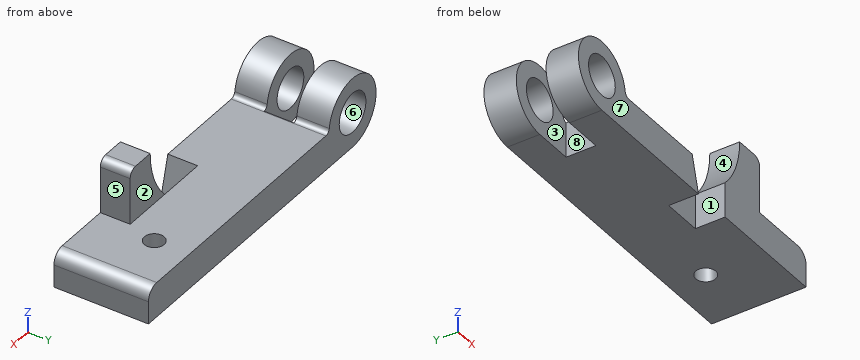
from build123d import *

# Parameters (mm, degrees)
F0_R          = 12.7
F1_DEPTH      = 30.1625
F2_R          = 6.35
F2_W          = 50.010991877
F2_H          = 18.9992
F3_DEPTH      = 22.353
F3_DEPTH_BACK = 25.4
F5_DEPTH      = 19.05
F7_DEPTH      = 19.05
F8_R          = 5.08
F9_R          = 7.874
F10_R         = 3.302


with BuildPart() as f1:
    # F0 (on Front) → F1 (new body, symmetric)
    with BuildSketch(Plane.XZ):
        with BuildLine():
            Line((194.2084, 0), (22.352, 0))
            ThreePointArc((22.352, 0), (-15.8052507731, 15.8052507731), (0, -22.352))
            Line((0, -22.352), (194.2084, -22.352))
            Line((194.2084, -22.352), (194.2084, 0))
        make_face()
        Circle(F0_R, mode=Mode.SUBTRACT)
    extrude(amount=F1_DEPTH, both=True)

    # F2 (on Top) → F3 (cut, two sides)
    with BuildSketch(Plane.XY) as f3_sk:
        with Locations((155.3464, 7.8105)):
            Circle(F2_R)
        Rectangle(F2_W, F2_H)
    extrude(amount=-F3_DEPTH, mode=Mode.SUBTRACT)
    extrude(f3_sk.sketch, amount=F3_DEPTH_BACK, mode=Mode.SUBTRACT)

    # F4 (on face) → F5 (cut)
    with BuildSketch(Plane.XZ.offset(30.1625)):
        Polygon((117.2464, -22.352), (117.2464, 0), (85.852, 0), (91.8464, -22.352), align=None)
    extrude(amount=-F5_DEPTH, mode=Mode.SUBTRACT)

    # F6 (on face) → F7 (join)
    with BuildSketch(Plane.XZ.offset(30.1625)):
        with BuildLine():
            Line((117.2464, 0), (150.0886, 0))
            Line((150.0886, 0), (150.0886, 34.798))
            Line((150.0886, 34.798), (131.0386, 34.798))
            ThreePointArc((131.0386, 34.798), (127.4644153616, 16.0823576341), (117.2464, 0))
        make_face()
    extrude(amount=-F7_DEPTH)

    # F8
    f8_edges = [f1.edges().sort_by_distance(p)[0] for p in [
        (150.0886, -20.6375, 34.798),
    ]]
    fillet(f8_edges, radius=F8_R)

    # F9
    f9_edges = [f1.edges().sort_by_distance(p)[0] for p in [
        (194.2084, 0, 0),
    ]]
    fillet(f9_edges, radius=F9_R)

    # F10
    f10_edges = [f1.edges().sort_by_distance(p)[0] for p in [
        (22.352, -19.83105, 0),
    ]]
    fillet(f10_edges, radius=F10_R)


solid = f1.part
The listing builds one solid part. Answer for the finished solid, in the listing's coordinates (mm). Face numbers are marked on the shaded views. A direction names the side the tool comes from. Round coordinates to 2 decimals unless told otherwise and drop trailing zeros. Write each loop counter-clockwise with the first axis right and the second up, starting at its lowest first coordinate (ties: lowest second). Pieces come first, ordered by that corner, then holes. Notation, with made-up numbers: (75.5, 64) - (130.5, 64) arc R20 cw to (130.5, 97) - close; hole circle Ø2 at (65, 34.25). An arc over 180 degrees is marked (long way). Use a Markdown table: item, result. Add a question column.
1. A tool of negligible diameter and unlimited length cuts with its end or side. For the marked faces 1, 2, 3, 4 and 5, from which of +Z, -Z, +X, -X, +Y, -Y can it reach the whole face along a straight path? Write none if from no direction.
2. The part is cut by section A-A (z = -3). Write down the section's boundary in (x, y).
3. For a pull along Y with two mould halves and no side action, classify the marked faces 6, 7 and 8 as +Y half, -Y half, draft (parallel to the pull), parting line (faces both ways), or undercut.
4. The part is cut by section D-D (x = 155). Write down the section's boundary in (y, z), and give its area (3 significant figures).
5. The part is cut by section B-B (y = 26). Write down the section's boundary in (x, z), and give its area (3 significant figures).
6. The part is cut by section C-C (z = 16). Write down the section's boundary in (x, y), and give its area (3 significant figures).
7. Flat-ended cylindrical pins translate along their axes: P1, Ø1, axis at x = 62, y = -15, coming from the +Z side; P2, Ø5.5, axis at y = -22.5, z = -11, coming from the -X side; P3, Ø18, axis at x = 97, z = -13, coming from the -Y side; P4, Ø15, axis at y = 3.5, z = -11.5, coming from the -X side. Find the tip coordinate at first contact, or state that the pin passes through.
8. Consider line 1 (Z direction, x = 0, y = -14.5); line 2 (Y direction, x = 149, z = 13); line 3 (Y direction, x = 91, z = -3). Determine where each line is inside the solid, lowest interval first.
Reported:
| question | item | result |
|---|---|---|
| 1 | face 1 | +Z, -Z, -Y |
| 1 | face 2 | +Z, +X, +Y |
| 1 | face 3 | +Z, -Z, -X |
| 1 | face 4 | +Z, +Y, -Y |
| 1 | face 5 | +Z, +X, +Y, -Y |
| 2 | outline | (-22.15, -30.16) - (-12.34, -30.16) - (-12.34, -9.5) - (-22.15, -9.5) - close; (-22.15, 9.5) - (-12.34, 9.5) - (-12.34, 30.16) - (-22.15, 30.16) - close; (12.34, -30.16) - (86.66, -30.16) - (86.66, -11.11) - (117.25, -11.11) - (117.25, -30.16) - (192.52, -30.16) - (192.52, 30.16) - (12.34, 30.16) - (12.34, 9.5) - (25.01, 9.5) - (25.01, -9.5) - (12.34, -9.5) - close; hole circle Ø12.7 at (155.35, 7.81) |
| 3 | face 6 | draft |
| 3 | face 7 | -Y half |
| 3 | face 8 | undercut |
| 4 | outline | (-30.16, -22.35) - (1.47, -22.35) - (1.47, 0) - (-30.16, 0) - close; (14.15, -22.35) - (30.16, -22.35) - (30.16, 0) - (14.15, 0) - close |
| 4 | area | 1,060 mm^2 |
| 5 | outline | (0, -22.35) - (194.21, -22.35) - (194.21, -7.87) arc R7.87 ccw to (186.33, 0) - (25.44, 0) arc R3.3 cw to (22.17, 2.88) arc R22.35 ccw (long way) to start; hole circle Ø25.4 at (0, 0) |
| 5 | area | 5,000 mm^2 |
| 6 | outline | (-15.61, -30.16) - (15.61, -30.16) - (15.61, -9.5) - (-15.61, -9.5) - close; (-15.61, 9.5) - (15.61, 9.5) - (15.61, 30.16) - (-15.61, 30.16) - close; (127.43, -30.16) - (150.09, -30.16) - (150.09, -11.11) - (127.43, -11.11) - close |
| 6 | area | 1,720 mm^2 |
| 7 | P1 | z = 0 |
| 7 | P2 | x = -20.77 |
| 7 | P3 | y = -30.16 |
| 7 | P4 | x = -21.23 |
| 8 | line 1 | -22.35 to -12.7, 12.7 to 22.35 |
| 8 | line 2 | -30.16 to -11.11 |
| 8 | line 3 | -11.11 to 30.16 |
